from build123d import *

# Parameters (mm, degrees)
EXTRUDE_1_DEPTH = 4


with BuildPart() as part:
    # 草图1 → 凸台-拉伸1 (new body)
    with BuildSketch(Plane.XY):
        Polygon((-39, 90), (-39, -46), (39, -46), (39, 90), (27.5, 90), (27.5, 86), (28.85, 86), (28.85, 83.3), (27.5, 83.3), (27.5, 81.3), (24.5, 81.3), (24.5, 83.3), (23.15, 83.3), (23.15, 86), (24.5, 86), (24.5, 90), (17, 90), (17, 94), (9, 94), (9, 90), (1.5, 90), (1.5, 86), (2.85, 86), (2.85, 83.3), (1.5, 83.3), (1.5, 81.3), (-1.5, 81.3), (-1.5, 83.3), (-2.85, 83.3), (-2.85, 86), (-1.5, 86), (-1.5, 90), (-9, 90), (-9, 94), (-17, 94), (-17, 90), (-24.5, 90), (-24.5, 86), (-23.15, 86), (-23.15, 83.3), (-24.5, 83.3), (-24.5, 81.3), (-27.5, 81.3), (-27.5, 83.3), (-28.85, 83.3), (-28.85, 86), (-27.5, 86), (-27.5, 90), align=None)
    extrude(amount=EXTRUDE_1_DEPTH)


solid = part.part
Source: CAD feature listing. Evaluate the final solid. Frame: model axes, mm. A direction names the side the tool comes from. Coordinates: 2 decimals unless noted, no trailing zeros. Write each question's results on one line, items separated by ' | '. Start each with the question number.
1. Reachability of faces 4 (the face through (-2.85, 85, 2)), 5 (the face through (-1, 25, 4)), 6 (the face through (-1, 25, 0)), 7 (the face through (27.5, 88, 2)), 8 (the face through (-33, 90, 2)) from +Z, -Z, +X, -X, +Y, -Y: full face, straight path, thin tool, end or side. Return the list, or none.
2. Draft query along X for faces 1 (the face through (17, 92, 2)), 2 (the face through (28.85, 85, 2)), 3 (the face through (33, 90, 2)). Return one class per face: +X half, -X half, draft (parallel to the pull), parting line (faces both ways), or undercut.
3. Material intervals for L1, parallel to X at y = 82.5, z = 3.8; L2, parallel to Y at x = -5.5, z = 2.95, sorted ascending.
4. Pin query (flat end, axial travel): pin 1 (1.2 mm diameter, centred on x = 32.5, z = 1.5, fed in from +Y); pin 2 (1.5 mm diameter, centred on x = -25.5, z = 3, fed in from +Y); pin 3 (1.2 mm diameter, centred on y = 91.5, z = 2.5, fed in from +X). Return the tip coordinate at first contact, or that it passes through.
Solution:
1) face 4: +Z, -Z | face 5: +Z, +X, -X, +Y, -Y | face 6: -Z, +X, -X, +Y, -Y | face 7: +Z, -Z, +Y | face 8: +Z, -Z, -X, +Y
2) face 1: +X half | face 2: undercut | face 3: draft
3) L1: -39 to -27.5, -24.5 to -1.5, 1.5 to 24.5, 27.5 to 39 | L2: -46 to 90
4) pin 1: y = 90 | pin 2: y = 81.3 | pin 3: x = 17
